For this review, take the finished solid that the model builds, in its own axes (mm). Give positions to 0.01 mm unless a question says otherwise; leave off trailing zeros. Write each loop counter-clockwise with the first axis right and the second up, starting at its lowest first coordinate (ties: lowest second). Pieces come first, ordered by that corner, then holes. Notation, with made-up numbers: (-35.5, -1.5) -> (9.5, -1.5) arc R19 ccw to (9.5, 27.5) -> close; hole circle Ø6 at (0.5, -12). An arc over 180 degrees is marked (long way). Write item = value, one per line.
```python
from build123d import *

# Parameters (mm, degrees)
F0_R     = 34.29
F1_DEPTH = 558.8
F2_R     = 46.99
F2_R_2   = 34.29
F3_DEPTH = 16.764
F4_R     = 34.29
F5_DEPTH = 241.3
F7_DEPTH = 38.354
F9_D     = 60.96


with BuildPart() as f1:
    # F0 (on Top) → F1 (new body)
    with BuildSketch(Plane.XY):
        with Locations((-27.8679728508, 21.5611346066)):
            Circle(F0_R)
    extrude(amount=F1_DEPTH)

    # F2 (on face) → F3 (join)
    with BuildSketch(Plane(origin=(0, 0, 0), x_dir=(1, 0, 0), z_dir=(0, 0, -1))):
        with Locations((-27.8679728508, -21.5611346066)):
            Circle(F2_R)
        with Locations((-27.8679728508, -21.5611346066)):
            Circle(F2_R_2, mode=Mode.SUBTRACT)
    extrude(amount=-F3_DEPTH)

    # F4 (on face) → F5 (join)
    with BuildSketch(Plane(origin=(0, 0, 0), x_dir=(1, 0, 0), z_dir=(0, 0, -1))):
        with Locations((-27.8679728508, -21.5611346066)):
            Circle(F4_R)
    extrude(amount=F5_DEPTH)

    # F6 (on face) → F7 (join)
    with BuildSketch(Plane(origin=(0, 0, -241.3), x_dir=(1, 0, 0), z_dir=(0, 0, -1))):
        with BuildLine():
            Line((5.7768958027, -26.0717726025), (5.7768958027, -14.9409447837))
            Line((5.7768958027, -14.9409447837), (-61.5128415043, -14.9409447837))
            ThreePointArc((-61.5128415043, -14.9409447837), (-61.702868113, -15.9930144037), (-61.86000493, -17.0504966107))
            Line((-61.86000493, -17.0504966107), (-61.86000493, -26.0717726025))
            Line((-61.86000493, -26.0717726025), (5.7768958027, -26.0717726025))
        make_face()
    extrude(amount=-F7_DEPTH)

    # F9 (through all)
    with Locations(Plane(origin=(0, 0, -241.3), x_dir=(1, 0, 0), z_dir=(0, 0, -1))):
        with Locations((-27.8679728508, -21.5611346066)):
            Hole(F9_D / 2)


solid = f1.part
```
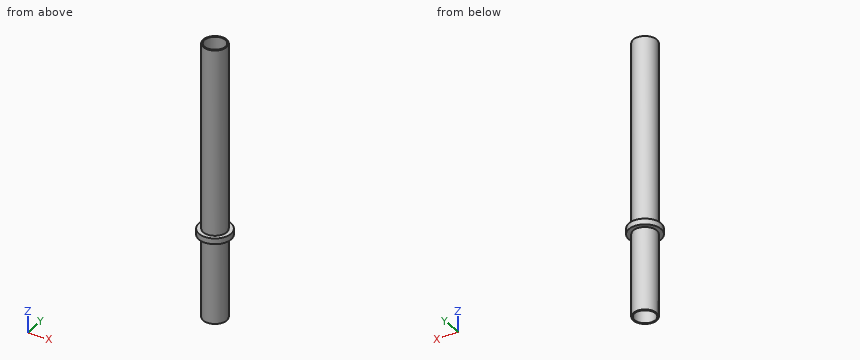
(1) Take a section at B-B (x = -48.5). Write out the cut boundary in (y, z), plus the area to 3 significant figures.
Answers below:
outline = (-20.66, 0) -> (-5.83, 0) -> (-5.83, -241.3) -> (-0.87, -241.3) -> (-0.87, 558.8) -> (-5.83, 558.8) -> (-5.83, 16.76) -> (-20.66, 16.76) -> close; (44, -241.3) -> (48.95, -241.3) -> (48.95, 0) -> (63.78, 0) -> (63.78, 16.76) -> (48.95, 16.76) -> (48.95, 558.8) -> (44, 558.8) -> close
area = 8,420 mm^2
(2) Take a section at A-A (y = 41.5). Write out the cut boundary in (x, z), plus the area to 3 significant figures.
Answers below:
outline = (-70.42, 0) -> (-55.77, 0) -> (-55.77, -241.3) -> (-50.92, -241.3) -> (-50.92, 558.8) -> (-55.77, 558.8) -> (-55.77, 16.76) -> (-70.42, 16.76) -> close; (-4.81, -241.3) -> (0.03, -241.3) -> (0.03, 0) -> (14.68, 0) -> (14.68, 16.76) -> (0.03, 16.76) -> (0.03, 558.8) -> (-4.81, 558.8) -> close
area = 8,240 mm^2
(3) Take a section at C-C (z = 345.5). Write out the cut boundary in (x, y).
Answers below:
outline = circle Ø68.58 at (-27.87, 21.56); hole circle Ø60.96 at (-27.87, 21.56)
(4) To check wall thickness, follow probe 1 along X at (y, z) = (18.5, 486); probe 2 along X at (y, z) = (46.5, -186); probe 3 along Y at (x, z) = (-24.5, 259). State the ranges of each line that lie inside material, in increasing order.
Answers below:
probe_1 = -62.02 to -58.19, 2.46 to 6.29
probe_2 = -51.4 to -45.39, -10.34 to -4.33
probe_3 = -12.56 to -8.73, 51.85 to 55.69
(5) For pin 1 (5 mm diameter, centred on y = 2, z = 199.5, fed in from +X); pin 2 (1.5 mm diameter, centred on x = -4, z = 370.5, fed in from +Y); pin 3 (8 mm diameter, centred on x = -7, y = 37.5, fed in from -Z); pin 4 (1 mm diameter, centred on x = -20.5, z = 350, fed in from -Y), all flat-tipped, find the tip position at first contact; note any pin that passes through.
Answers below:
pin_1 = 1.88
pin_2 = 46.89
pin_3 = through
pin_4 = -12.03
